Check sheet for the modelled part. Datum: model origin and axes. Units: mm. A direction names the side the tool comes from. Coordinates: 2 decimals unless noted, no trailing zeros. Loops run counter-clockwise (first coordinate to the right, second up) from the corner with the lowest first, then second, coordinate; pieces in that order, holes last.
```python
from build123d import *

# Parameters (mm, degrees)
F0_W     = 38.1
F0_H     = 71.4375
F1_DEPTH = 12.7
F2_T     = -1.5875
F3_R     = 1.27


with BuildPart() as f1:
    # F0 (on Top) → F1 (new body)
    with BuildSketch(Plane.XY):
        Rectangle(F0_W, F0_H)
    extrude(amount=F1_DEPTH)

    # F2
    f2_openings = [f1.faces().sort_by_distance(p)[0] for p in [
        (0, 0, 12.7),
    ]]
    offset(amount=F2_T, openings=f2_openings)

    # F3
    f3_edges = [f1.edges().sort_by_distance(p)[0] for p in [
        (-19.05, -35.71875, 6.35),
        (19.05, -35.71875, 6.35),
        (-19.05, 35.71875, 6.35),
        (19.05, 35.71875, 6.35),
    ]]
    fillet(f3_edges, radius=F3_R)


solid = f1.part
```
1) Scan lines: line 1 (X direction, y = 8, z = 7.75); line 2 (Y direction, x = 14, z = 11.75); line 3 (Z direction, x = 3.5, y = 10). Record each from-to range of solid material in increasing order.
Answer sheet:
line 1: x = -19.05 to -17.46, 17.46 to 19.05
line 2: y = -35.72 to -34.13, 34.13 to 35.72
line 3: z = 0 to 1.59
2) Section check C-C on x = 11. Enter the section's corners in (y, z), plus the area to 3 significant figures.
Answer sheet:
outline: (-35.72, 0) - (35.72, 0) - (35.72, 12.7) - (34.13, 12.7) - (34.13, 1.59) - (-34.13, 1.59) - (-34.13, 12.7) - (-35.72, 12.7) - close
area: 149 mm2
3) Set-up check for faces 4 (the flat face through (19.05, 0, 6)), 5 (the flat face through (0, 34.131, 7)): record each of +Z, -Z, +X, -X, +Y, -Y from which the full face is reachable in a straight line by a thin tool's end or side.
Answer sheet:
face 4: +Z, -Z, +X, +Y, -Y
face 5: +Z
4) Section check A-A on z = 3.5. Enter the section's corners in (x, y), plus the area to 3 significant figures.
Answer sheet:
outline: (-19.05, -34.45) arc R1.27 ccw to (-17.78, -35.72) - (17.78, -35.72) arc R1.27 ccw to (19.05, -34.45) - (19.05, 34.45) arc R1.27 ccw to (17.78, 35.72) - (-17.78, 35.72) arc R1.27 ccw to (-19.05, 34.45) - close; hole (-17.46, -34.13) - (17.46, -34.13) - (17.46, 34.13) - (-17.46, 34.13) - close
area: 336 mm2
5) Mould release check, pull along X, two halves, no side actions. Record for faces 1 (the flat face through (-19.05, 0, 6)), 2 (the cylindrical face through (18.688, 35.337, 6.439)), 3 (the flat face through (0, -34.131, 7)): +X half, -X half, draft (parallel to the pull), parting line (faces both ways), or undercut.
Answer sheet:
face 1: -X half
face 2: +X half
face 3: undercut
6) Section check B-B on y = 23. Enter the section's corners in (x, z), plus the area to 3 significant figures.
Answer sheet:
outline: (-19.05, 0) - (19.05, 0) - (19.05, 12.7) - (17.46, 12.7) - (17.46, 1.59) - (-17.46, 1.59) - (-17.46, 12.7) - (-19.05, 12.7) - close
area: 95.8 mm2
